Model file for the job. Use its own axes, mm. A direction names the side the tool comes from. Round coordinates to 2 decimals unless told otherwise and drop trailing zeros. Loops run counter-clockwise (first coordinate to the right, second up) from the corner with the lowest first, then second, coordinate; pieces in that order, holes last. Notation, with made-up numbers: (29, 4.25) -> (75, 4.25) arc R23 ccw to (75, 42.25) -> close; hole circle Ø8 at (42.25, 62). An arc over 180 degrees is marked (long way). Use a Markdown table: item, result.
from build123d import *

# Parameters (mm, degrees)
SKETCH2_R          = 15.875
CUT_EXTRUDE1_DEPTH = 77.2
FILLET2_R          = 10.16
FILLET3_R          = 10.16


with BuildPart() as part:
    # Sketch1 → Revolve2 (revolve)
    with BuildSketch(Plane.XY):
        Polygon((-38.1, -0.729526652), (-38.1, 24.670473348), (-12.7, 24.670473348), (-12.7, 75.470473348), (-38.1, 75.470473348), (-38.1, 100.870473348), (38.1, 100.870473348), (38.1, 75.470473348), (12.7, 75.470473348), (12.7, 24.670473348), (38.1, 24.670473348), (38.1, -0.729526652), align=None)
    revolve(axis=Axis((-38.1, -0.729526652, 0), (1, 0, 0)))

    # Sketch2 → Cut-Extrude1 (cut, through all)
    with BuildSketch(Plane(origin=(38.1, 0, 0), x_dir=(0, 0, -1), z_dir=(1, 0, 0))):
        Circle(SKETCH2_R)
    extrude(amount=-CUT_EXTRUDE1_DEPTH, mode=Mode.SUBTRACT)

    # Fillet2
    fillet2_edges = [part.edges().sort_by_distance(p)[0] for p in [
        (38.1, -102.329526652, 0),
    ]]
    fillet(fillet2_edges, radius=FILLET2_R)

    # Fillet3
    fillet3_edges = [part.edges().sort_by_distance(p)[0] for p in [
        (-38.1, -102.329526652, 0),
    ]]
    fillet(fillet3_edges, radius=FILLET3_R)


solid = part.part
Q1. Band-saw the part on C-C, the plane x = -0.5. Give the cut face in (y, z) (3 decimals).
Results list:
| item | result |
|---|---|
| outline | circle Ø203.2 at (-0.73, 0); hole circle Ø31.75 at (0, 0) |
Q2. Band-saw the part on B-B, the plane z = 0. Give the cut face in (x, y) (3 decimals).
Results list:
| item | result |
|---|---|
| outline | (-38.1, -92.17) arc R10.16 ccw to (-27.94, -102.33) -> (27.94, -102.33) arc R10.16 ccw to (38.1, -92.17) -> (38.1, -76.93) -> (12.7, -76.93) -> (12.7, -26.13) -> (38.1, -26.13) -> (38.1, -15.875) -> (-38.1, -15.875) -> (-38.1, -26.13) -> (-12.7, -26.13) -> (-12.7, -76.93) -> (-38.1, -76.93) -> close; (-38.1, 15.875) -> (38.1, 15.875) -> (38.1, 24.67) -> (12.7, 24.67) -> (12.7, 75.47) -> (38.1, 75.47) -> (38.1, 90.71) arc R10.16 ccw to (27.94, 100.87) -> (-27.94, 100.87) arc R10.16 ccw to (-38.1, 90.71) -> (-38.1, 75.47) -> (-12.7, 75.47) -> (-12.7, 24.67) -> (-38.1, 24.67) -> close |
Q3. Band-saw the part on A-A, the plane x = -20. Give the cut face in (y, z) (3 decimals).
Results list:
| item | result |
|---|---|
| outline | circle Ø203.2 at (-0.73, 0); circle Ø50.8 at (-0.73, 0); hole circle Ø152.4 at (-0.73, 0); hole circle Ø31.75 at (0, 0) |
Q4. Drill centre lines: L1, parallel to Y at x = 34, z = -12; L2, parallel to Z at x = 18, y = -24; L3, parallel to Z at x = 14, y = 6.5. Where is each one in solid material? Low to high. Write a range as from..to.
Results list:
| item | result |
|---|---|
| L1 | y = -99.6..-75.98, -23.12..-10.39, 10.39..21.66, 74.52..98.14 |
| L2 | z = -98.9..-72.56, -10.18..10.18, 72.56..98.9 |
| L3 | z = -101.34..-75.86, -24.35..-14.48, 14.48..24.35, 75.86..101.34 |
Q5. Flat gauge pins, fed straight in: pin 1 (2 mm diameter, centred on x = 6, y = -31, fed in from -Z); pin 2 (1.5 mm diameter, centred on x = 20.5, z = -70, fed in from +Y); pin 3 (5 mm diameter, centred on x = -3, y = 18, fed in from +Z). Where does each tip first touch, or does it go through?
Results list:
| item | result |
|---|---|
| pin 1 | stops at z = -97.29 |
| pin 2 | stops at y = 73.61 |
| pin 3 | stops at z = 100.3 |
Q6. Pull direction Z, two halves, no side cores. Call faces 1 (the face through (38.1, -12, -11)), 2 (the face through (25.222, -61.199, -46.367)), 3 (the face through (0.391, -13.956, 100.735)): released by +Z, released by -Z, zero draft, split by the parting line, or undercut.
Results list:
| item | result |
|---|---|
| face 1 | zero draft |
| face 2 | undercut |
| face 3 | split by the parting line |
Q7. Tool access for faces 4 (the face through (25.578, -4.036, 25.184)), 5 (the face through (-12.7, -34, 1)), 6 (the face through (-38.1, -12, -11)): list every direction of +Z, -Z, +X, -X, +Y, -Y with a clear straight run to the whole face (end or side of a thin tool).
Results list:
| item | result |
|---|---|
| face 4 | +X |
| face 5 | -X |
| face 6 | +Z, -Z, -X, +Y, -Y |
